Autodesk Inventor part; units mm, degrees
ref_plane "Work Plane4" through (0, 10, 0) normal (0, 1, 0) x (-1, 0, 0)
ref_plane "YZ Plane" through (0, 0, 0) normal (1, 0, 0) x (0, 1, 0)
ref_plane "XY Plane" through (0, 0, 0) normal (0, 0, 1) x (1, 0, 0)
sketch "Sketch9" plane through (0, 0, 0) normal (1, 0, 0) x (0, 1, 0)
  circle A0 centre (0, 0) radius 10
  circle A1 centre (0, 0) radius 3.4
  dimension "d31" = 20
  dimension "d32" = 6.8
extrude "Extrusion7" add sketch "Sketch9" along normal blind 9
sketch "Sketch10" plane through (9, 0, 0) normal (1, 0, 0) x (0, 0, -1)
  circle A0 centre (0, 0) radius 7.5
  dimension "d35" = 15
extrude "Extrusion8" cut sketch "Sketch10" against normal blind 0.5
ref_plane "Work Plane3" through (0, 5.5, 0) normal (0, 1, 0) x (-1, 0, 0)
sketch "Sketch11" plane through (0, 5.5, 0) normal (0, 1, 0) x (-1, 0, 0)
  line L0 (0, 0) -> (-9, 0) construction
  line L1 (-9, 10) -> (-9, -10) construction
  line L2 (-7.9064, 0) -> (-6.2032, 2.95)
  line L3 (-6.2032, 2.95) -> (-2.7968, 2.95)
  line L4 (-2.7968, 2.95) -> (-1.0936, 0)
  line L5 (-1.0936, 0) -> (-2.7968, -2.95)
  line L6 (-2.7968, -2.95) -> (-6.2032, -2.95)
  line L7 (-6.2032, -2.95) -> (-7.9064, 0)
  line L8 (-6.2032, 2.95) -> (-9, 2.95)
  line L9 (-9, 2.95) -> (-9, -2.95)
  line L10 (-9, -2.95) -> (-6.2032, -2.95)
  point P0 (-4.5, 0)
  dimension "d39" = 5.9
extrude "Extrusion9" cut sketch "Sketch11" along normal mid plane 3
ref_plane "Work Plane4" through (0, 10, 0) normal (0, 1, 0) x (-1, 0, 0)
sketch "Sketch12" plane through (0, 10, 0) normal (0, 1, 0) x (-1, 0, 0)
  line L0 (-2.7968, 2.95) -> (-1.0936, 0) construction
  line L1 (-1.9452, 1.475) -> (-5.8393, -0.7732) construction
  line L2 (-1.0936, 0) -> (-2.7968, -2.95) construction
  line L3 (-1.9452, -1.475) -> (-5.6209, 0.6472) construction
  circle A0 centre (-4.5, 0) radius 2.95 construction
  point P0 (0, 0)
hole "Hole2" at (4.5, 10, 0) direction (0, -1, 0) diameter 3.1 depth 10
mirror "Mirror2" about plane through (0, 0, 0) normal (0, 1, 0) of "Extrusion9", "Hole2"
properties part number "Swivel Joint Axle Lock Grub Screw"
The listing builds one solid part. Answer for the finished solid, in the listing's coordinates (mm). A direction names the side the tool comes from. Give positions to 0.01 mm unless a question says otherwise; leave off trailing zeros. Write each loop counter-clockwise with the first axis right and the second up, starting at its lowest first coordinate (ties: lowest second). Pieces come first, ordered by that corner, then holes. Notation, with made-up numbers: (3, 54.25) -> (51, 54.25) arc R21 ccw to (51, 67.25) -> close; hole circle Ø10 at (-39.5, -11). An arc over 180 degrees is marked (long way). Write item = value, one per line. Start each with the question number.
1) The part is cut by section C-C, the plane x = 4.5. Determine the outline of the cut face in (y, z), and give its area (3 significant figures).
2) The part is cut by section D-D, the plane z = -6.75. Determine the outline of the cut face in (x, y).
3) Determine the mould class of faces 1 (the face through (6, 7, 1)), 2 (the face through (2.963, 8.479, -0.202)), 3 (the face through (1.96, 5.48, 1.5)) for opening direction X: +X half, -X half, draft (parallel to the pull), parting line (faces both ways), or undercut.
4) Straight lines are drawn through the part: line 1 along Y through (x, z) = (5.5, 1.5); line 2 along Z through (x, y) = (7.5, 1.5); line 3 along X through (y, z) = (6.5, -3). For each, find the intervals that lie inside material, in ascending order.
5) The part is cut by section B-B, the plane x = 7.75. Determine the outline of the cut face in (y, z), and give its area (3 significant figures).
6) Which of the six approach directions +Z, -Z, +X, -X, +Y, -Y give full straight-line access (tool end or side, diameter ignored) to faces 4 (the face through (0, 4, 0)), 5 (the face through (6.5, 4, 0))?
7) Each of these flat-tipped pins is pushed along its axis until it touches: pin 1 (3 mm diameter, centred on x = 6.5, y = 6.5, fed in from -Z); pin 2 (2 mm diameter, centred on x = 3, z = 2, fed in from -Y); pin 3 (5 mm diameter, centred on x = 6.5, z = 6.5, fed in from +Y). Where does it stop, or does it pass through?
8) The part is cut by section A-A, the plane y = 0. Determine the outline of the cut face in (x, z), and give its area (3 significant figures).
Solutions:
q1.outline = (-9.88, -1.55) arc R10 ccw to (9.88, -1.55) -> (7, -1.55) -> (7, -2.95) -> (4, -2.95) -> (4, -1.55) -> (3.03, -1.55) arc R3.4 cw to (-3.03, -1.55) -> (-4, -1.55) -> (-4, -2.95) -> (-7, -2.95) -> (-7, -1.55) -> close; (-9.88, 1.55) -> (-7, 1.55) -> (-7, 2.95) -> (-4, 2.95) -> (-4, 1.55) -> (-3.03, 1.55) arc R3.4 cw to (3.03, 1.55) -> (4, 1.55) -> (4, 2.95) -> (7, 2.95) -> (7, 1.55) -> (9.88, 1.55) arc R10 ccw to start
q1.area = 220 mm²
q2.outline = (0, -7.38) -> (9, -7.38) -> (9, -3.27) -> (8.5, -3.27) -> (8.5, 3.27) -> (9, 3.27) -> (9, 7.38) -> (0, 7.38) -> close
q3.face_1 = draft
q3.face_2 = undercut
q3.face_3 = +X half
q4.line_1 = -9.89 to -7, -4 to -3.05, 3.05 to 4, 7 to 9.89
q4.line_2 = -9.89 to -3.05, 3.05 to 9.89
q4.line_3 = 0 to 8.5
q5.outline = circle Ø20 at (0, 0); hole (-7, -2.95) -> (-4, -2.95) -> (-4, 2.95) -> (-7, 2.95) -> close; hole circle Ø6.8 at (0, 0); hole (4, -2.95) -> (7, -2.95) -> (7, 2.95) -> (4, 2.95) -> close
q5.area = 242 mm²
q6.face_4 = +Z, -Z, -X, +Y, -Y
q6.face_5 = +X
q7.pin_1 = -8.66
q7.pin_2 = -9.95
q7.pin_3 = 9.17
q8.outline = (0, -10) -> (9, -10) -> (9, -7.5) -> (8.5, -7.5) -> (8.5, -3.4) -> (0, -3.4) -> close; (0, 3.4) -> (8.5, 3.4) -> (8.5, 7.5) -> (9, 7.5) -> (9, 10) -> (0, 10) -> close
q8.area = 115 mm²
